For this review, take the finished solid that the model builds, in its own axes (mm). A direction names the side the tool comes from. Give positions to 0.01 mm unless a question says otherwise; leave off trailing zeros. Order: outer loops, then holes, each group sorted by start corner. A loop starts at its lowest first (then second) coordinate and runs counter-clockwise, first axis right, second up.
Item 1: Consider section B-B (y = 4.75). Give the boundary of the cut face in (x, z).
Item 2: The part is to be moulded in two halves that separate along Z. For faces 4 (the flat face through (8.47, 5.07, -6.95)), 5 (the flat face through (0.4, 4.9, 10.1)), 6 (the flat face through (-4, 4, -7.1)), say which applies: released by +Z, released by -Z, zero draft, split by the parting line, or undercut.
Item 3: Machinability: for faces 1 (the flat face through (6, 5, 0)), 2 (the cylindrical face through (5.87, 5.07, -9.79)), 3 (the flat face through (2, 5, 0)), which of the approach directions +Z, -Z, +X, -X, +Y, -Y give a long, thin tool a straight path to every point of the face, cutting with its end or side? Answer none if there is none.
Item 4: Consider section C-C (x = 6.25). Give the boundary of the cut face in (y, z).
Item 5: Consider section D-D (z = -8.25). Give the boundary of the cut face in (x, y), plus the area to 3 significant figures.
Item 6: Consider section A-A (x = -2). Give the boundary of the cut face in (y, z).
Item 7: For probe 1 along Z at (x, y) = (-2.25, 7.5); probe 2 along X at (y, z) = (7.5, -4); probe 3 along Y at (x, z) = (-2.5, 9), list the stretches that pass through material, from the lowest coordinate up.
Item 8: For P1, Ø1, axis at x = 6.5, z = -5, coming from the -Y side; P2, Ø1.2, axis at x = 9, y = 4.5, coming from the -Z side; P3, Ø1, axis at x = 8.5, y = 5.5, coming from the -Z side; P4, Ø3, axis at x = 9, y = 6.5, coming from the +Z side, all flat-tipped, find the tip position at first contact; note any pin that passes through.
```python
from build123d import *

# Parameters (mm, degrees)
BOSS_EXTRUDE1_DEPTH     = 10
CUT_EXTRUDE1_DEPTH      = 21.780760333
CUT_EXTRUDE1_DEPTH_BACK = 21.780760333
BOSS_EXTRUDE2_DEPTH     = 10
FILLET1_R               = 3


with BuildPart() as part:
    # Sketch1 → Boss-Extrude1 (new body)
    with BuildSketch(Plane(origin=(0, 0, 0), x_dir=(1, 0, 0), z_dir=(0, 1, 0))):
        Polygon((-6, -10.1), (6, -10.1), (6, 10.1), (-6, 10.1), (-6, 7.1), (2, 7.1), (2, -7.1), (-6, -7.1), align=None)
    extrude(amount=BOSS_EXTRUDE1_DEPTH)

    # Sketch2 → Cut-Extrude1 (cut, two sides: drawn at the far end of the back side and taken through both)
    with BuildSketch(Plane.XY.offset(-7.1).offset(-CUT_EXTRUDE1_DEPTH_BACK)):
        with BuildLine():
            ThreePointArc((-3.280624847, 6.600781059), (-3.600781059, 3.719375153), (-0.719375153, 3.399218941))
            Line((-0.719375153, 3.399218941), (-3.280624847, 6.600781059))
        make_face()
        with BuildLine():
            Line((-3.280624847, 6.600781059), (-0.719375153, 3.399218941))
            ThreePointArc((-0.719375153, 3.399218941), (-0.152328366, 4.111963102), (0.05, 5))
            ThreePointArc((0.05, 5), (-1.111963102, 6.847671634), (-3.280624847, 6.600781059))
        make_face()
    extrude(amount=CUT_EXTRUDE1_DEPTH + CUT_EXTRUDE1_DEPTH_BACK, mode=Mode.SUBTRACT)

    # Sketch3 → Boss-Extrude2 (add)
    with BuildSketch(Plane(origin=(0, 10, 0), x_dir=(1, 0, 0), z_dir=(0, 1, 0))):
        Polygon((10, 5), (6, 10.1), (6, 5), align=None)
        Polygon((6, -10.1), (10, -5), (6, -5), align=None)
    extrude(amount=-BOSS_EXTRUDE2_DEPTH)

    # Fillet1
    fillet1_edges = [part.edges().sort_by_distance(p)[0] for p in [
        (6, 5, -10.1),
        (6, 5, 10.1),
    ]]
    fillet(fillet1_edges, radius=FILLET1_R)


solid = part.part
```
Resolved:
1. outline: (-6, -10.1) - (-4.03, -10.1) - (-4.03, -7.1) - (-6, -7.1) - close; (-6, 7.1) - (-4.03, 7.1) - (-4.03, 10.1) - (-6, 10.1) - close; (0.03, -10.1) - (4.54, -10.1) arc R3 ccw to (6.9, -8.95) - (10, -5) - (6, -5) - (6, 5) - (10, 5) - (6.9, 8.95) arc R3 ccw to (4.54, 10.1) - (0.03, 10.1) - (0.03, 7.1) - (2, 7.1) - (2, -7.1) - (0.03, -7.1) - close
2. face 4: released by -Z
2. face 5: released by +Z
2. face 6: undercut
3. face 1: +X, +Y, -Y
3. face 2: -Z, +X, +Y, -Y
3. face 3: -X, +Y, -Y
4. outline: (0, -9.57) - (10, -9.57) - (10, -5) - (0, -5) - close; (0, 5) - (10, 5) - (10, 9.57) - (0, 9.57) - close
5. outline: (-6, 0) - (7.45, 0) - (7.45, 10) - (-6, 10) - close; hole circle Ø4.1 at (-2, 5)
5. area: 121 mm2
6. outline: (0, -10.1) - (2.95, -10.1) - (2.95, -7.1) - (0, -7.1) - close; (0, 7.1) - (2.95, 7.1) - (2.95, 10.1) - (0, 10.1) - close; (7.05, -10.1) - (10, -10.1) - (10, -7.1) - (7.05, -7.1) - close; (7.05, 7.1) - (10, 7.1) - (10, 10.1) - (7.05, 10.1) - close
7. probe 1: z = -10.1 to -7.1, 7.1 to 10.1
7. probe 2: x = 2 to 6
7. probe 3: y = 0 to 3.01, 6.99 to 10
8. P1: stops at y = 0
8. P2: stops at z = -7.04
8. P3: stops at z = -7.55
8. P4: stops at z = 8.19
